Print and shaded views of the part. All mm, measured from the part's lowest x, y and z. A direction names the side the tool comes from. Coordinates: 2 decimals unless noted, no trailing zeros. Loops run counter-clockwise (first coordinate to the right, second up) from the corner with the lowest first, then second, coordinate; pieces in that order, holes last. Notation, with made-up numbers: M 10,30.5 L 18,30.5 A13 cw 18,53.5 Z; hole C 6,87 d10. An arc over 180 degrees is marked long. Answer as a JSON object with one key per item and string values. Group by question number.
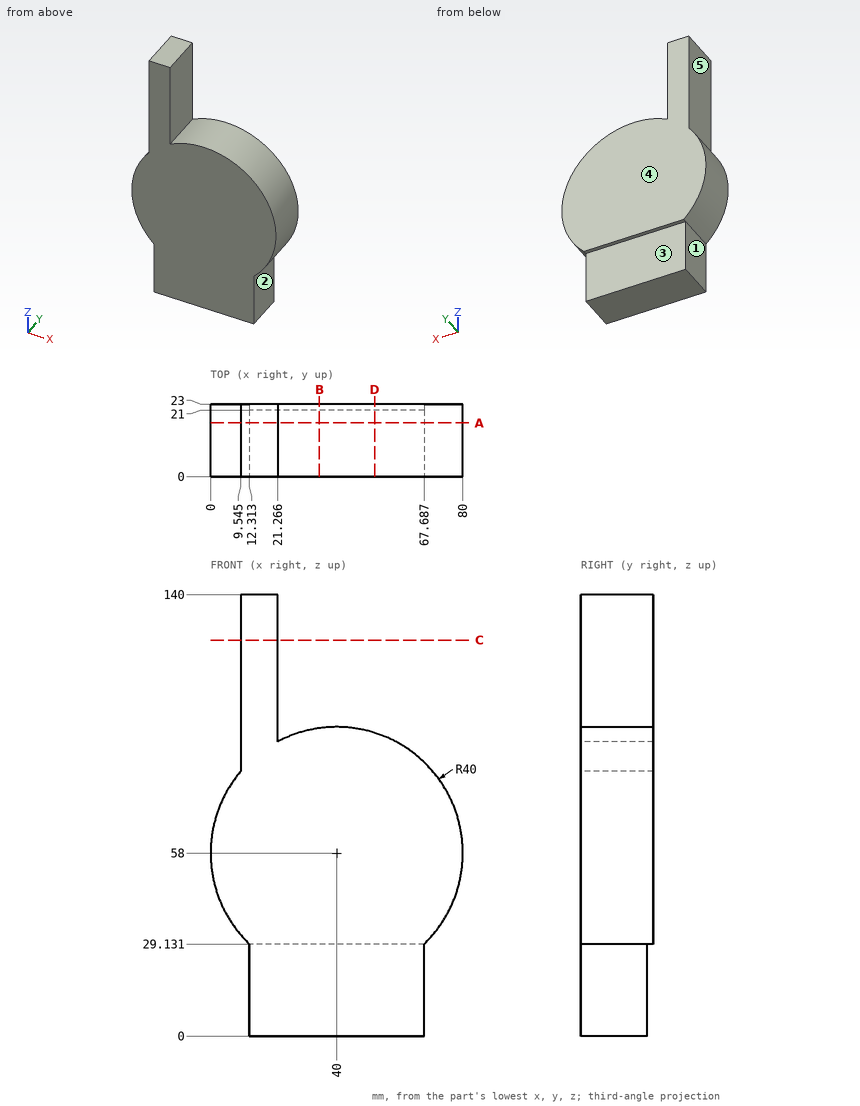
Item 1: Drill centre lines: L1, parallel to X at y = 10.75, z = 27.5; L2, parallel to Z at x = 41.5, y = 15; L3, parallel to X at y = 6, z = 129.5 (1 decimal). Where is each one in solid material? Low to high. Write a range as from..to.
Item 2: Slice it at D-D, the plane x = 52. Write the cut outline in (y, z), then the cut area to 3 significant figures.
Item 3: Pin check, flat tips, straight feed: pin 1 (5 mm diameter, centred on y = 11, z = 82, fed in from -X); pin 2 (10.5 mm diameter, centred on y = 12, z = 18, fed in from +X); pin 3 (6 mm diameter, centred on y = 12, z = 48, fed in from +X). Stop position of each tip, or through.
Item 4: Slice it at A-A, the plane y = 17. Write the cut outline in (x, z) (1 decimal), then the cut area to 3 significant figures.
Item 5: Tool access for the marked faces 1, 2, 3, 4 and 5: list every direction of +Z, -Z, +X, -X, +Y, -Y with a clear straight run to the whole face (end or side of a thin tool).
Item 6: Slice it at B-B, the plane x = 34.5. Write the cut outline in (y, z).
Item 7: Slice it at C-C, the plane z = 125.5. Write the cut outline in (x, y) (1 decimal).
Computed:
{
 "1": {"L1": "12.31..67.69", "L2": "0..97.97", "L3": "9.5..21.3"},
 "2": {"outline": "M 0,0 L 21,0 L 21,29.13 L 23,29.13 L 23,96.16 L 0,96.16 Z", "area": "2,150 mm2"},
 "3": {"pin 1": "x = 6.27", "pin 2": "x = 67.69", "pin 3": "x = 79.38"},
 "4": {"outline": "M 9.5,83.9 A40 ccw 12.3,29.1 L 12.3,0 L 67.7,0 L 67.7,29.1 A40 ccw 21.3,93.3 L 21.3,140 L 9.5,140 Z", "area": "6,810 mm2"},
 "5": {"face 1": "-Z, -X, +Y, -Y", "face 2": "-Z, +X, +Y, -Y", "face 3": "-Z, +X, -X, +Y", "face 4": "+Z, -Z, +X, -X, +Y", "face 5": "+Z, -X, +Y, -Y"},
 "6": {"outline": "M 0,0 L 21,0 L 21,29.13 L 23,29.13 L 23,97.62 L 0,97.62 Z"},
 "7": {"outline": "M 9.5,0 L 21.3,0 L 21.3,23 L 9.5,23 Z"}
}
